```python
from build123d import *

# Parameters (mm, degrees)
SKETCH1_W           = 26
SKETCH1_H           = 10.7
BOSS_EXTRUDE1_DEPTH = 6.85


with BuildPart() as part:
    # Sketch1 → Boss-Extrude1 (new body)
    with BuildSketch(Plane(origin=(0, 0, 0), x_dir=(1, 0, 0), z_dir=(0, 1, 0))):
        Rectangle(SKETCH1_W, SKETCH1_H)
    extrude(amount=BOSS_EXTRUDE1_DEPTH)

    # Sketch2 → section 0 of loft1
    with BuildSketch(Plane.ZY.offset(15.8), mode=Mode.PRIVATE) as loft1_s0:
        with BuildLine():
            Line((3.75, 1.425), (-3.75, 1.425))
            Line((-3.75, 1.425), (-3.75, 5.425))
            Line((-3.75, 5.425), (3.75, 5.425))
            Line((3.75, 5.425), (3.75, 1.425))
        make_face()
    # loft up to a face of the part (loft1)
    loft([loft1_s0.sketch, part.faces().sort_by_distance((-13, 3.425, 0))[0]])

    # Sketch4 → Loft2 section 0
    with BuildSketch(Plane.XY.offset(5.35)):
        with BuildLine():
            Line((13, 6.85), (3, 6.85))
            Line((3, 6.85), (3, 0))
            Line((3, 0), (13, 0))
            Line((13, 0), (13, 6.85))
        make_face()
    # Sketch3 → Loft2 section 1
    with BuildSketch(Plane.XY.offset(8.15)):
        with BuildLine():
            Line((4.25, 1.425), (11.75, 1.425))
            Line((11.75, 1.425), (11.75, 5.425))
            Line((11.75, 5.425), (4.25, 5.425))
            Line((4.25, 5.425), (4.25, 1.425))
        make_face()
    loft2 = loft()

    # Mirror1: Loft2 across plane
    add(loft2.mirror(Plane.XY))


solid = part.part
```
Input: part model. Units: mm. Frame: model coordinates. A direction names the side the tool comes from. Coordinates: 2 decimals unless noted, no trailing zeros. Loops run counter-clockwise (first coordinate to the right, second up) from the corner with the lowest first, then second, coordinate; pieces in that order, holes last.
Q1. Line query: line 1 along Z through (x, y) = (-7, 5.5); line 2 along X through (y, z) = (4.25, -6.5); line 3 along Z through (x, y) = (12, 3.5). Output: solid intervals per line, ascending.
Results are:
line 1: z = -5.35 to 5.35
line 2: x = 3.51 to 12.49
line 3: z = -7.59 to 7.59
Q2. Contact query for flat-ended pins moving along their axis: pin 1 (4 mm diameter, centred on x = -4.5, y = 4, fed in from -Z); pin 2 (2 mm diameter, centred on x = -9, y = 3, fed in from +Z). Output: stop coordinate, or through.
Results are:
pin 1: stops at z = -5.35
pin 2: stops at z = 5.35
Q3. Section A-A, the plane x = 0. Return the cut outline in (y, z), and give its area (3 significant figures).
Results are:
outline: (0, -5.35) - (6.85, -5.35) - (6.85, 5.35) - (0, 5.35) - close
area: 73.3 mm2
Q4. Set-up query: faces 1 (the flat face through (-5, 3, -5.35)), 2 (the flat face through (-5, 3, 5.35)), 3 (the flat face through (-15.8, 3, 0)). Return all of +Z, -Z, +X, -X, +Y, -Y with unobstructed straight access to the full face (end or side cutting, diameter ignored); none if empty.
Results are:
face 1: -Z, -X, +Y, -Y
face 2: +Z, -X, +Y, -Y
face 3: +Z, -Z, -X, +Y, -Y
